```python
from build123d import *

# Parameters (mm, degrees)
F0_R           = 35.367098
F1_DEPTH       = 22.86
F2_D           = 20
F2_CBORE_D     = 22
F2_CBORE_DEPTH = 6.6
F3_R           = 10.89761
F4_DEPTH       = 6.604
F5_R           = 10.16


with BuildPart() as f1:
    # F0 (on Top) → F1 (new body)
    with BuildSketch(Plane.XY):
        Circle(F0_R)
    extrude(amount=F1_DEPTH)

    # F2 (through all)
    with Locations(Plane(origin=(0, 0, 0), x_dir=(1, 0, 0), z_dir=(0, 0, -1))):
        with Locations((0, 0)):
            CounterBoreHole(F2_D / 2, F2_CBORE_D / 2, F2_CBORE_DEPTH)

    # F3 (on face) → F4 (cut)
    with BuildSketch(Plane.XY.offset(22.86)):
        Circle(F3_R)
    extrude(amount=-F4_DEPTH, mode=Mode.SUBTRACT)

    # F5
    f5_edges = [f1.edges().sort_by_distance(p)[0] for p in [
        (35.367098, 0, 11.43),
        (-35.367098, 0, 0),
        (-35.367098, 0, 22.86),
    ]]
    fillet(f5_edges, radius=F5_R)


solid = f1.part
```
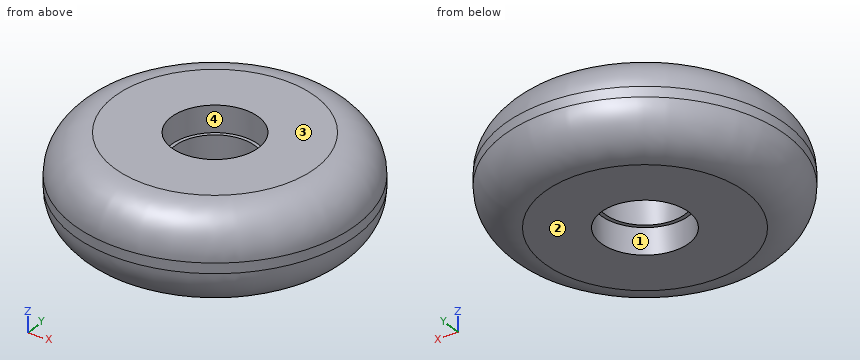
CAD build for the part. Positions are in the model's coordinates, mm. Face numbers are marked on the shaded views. A direction names the side the tool comes from. Coordinates: 2 decimals unless noted, no trailing zeros. Order: outer loops, then holes, each group sorted by start corner. A loop starts at its lowest first (then second) coordinate and runs counter-clockwise, first axis right, second up. Notation, with made-up numbers: (43, 76) - (63, 76) arc R8 cw to (63, 80) - close; hole circle Ø7 at (-7, 1.5). An arc over 180 degrees is marked (long way). Use a Markdown table: item, result. Add a question column.
(1) Saw through at A-A (x = 0). Give the cut face in (y, z), then the cut area to 3 significant figures.
(2) Saw through at D-D (z = 20.5). Give the cut face in (x, y).
(3) Drill centre lines: line 1 along Y through (x, z) = (0.5, 10.25); line 2 along Y through (x, z) = (0, 17.75); line 3 along X through (y, z) = (-7.5, 13). Where is each one in solid material? Low to high. Write a range as [from, to].
(4) Which spindle directions (+Z, -Z, +X, -X, +Y, -Y) get a long thin tool onto all of the face, cutting with end or side? Do the marked faces 3 and 4. Say none if no direction does.
(5) Saw through at C-C (z = 7.75). Give the cut face in (x, y).
(6) Pull direction Y, two halves, no side cores. Call the marked faces 1 and 2: +Y half, -Y half, draft (parallel to the pull), parting line (faces both ways), or undercut.
(7) Flat gauge pins, fed straight in: pin 1 (4 mm diameter, centred on y = -25.5, z = 14.5, fed in from +X); pin 2 (8 mm diameter, centred on y = -23.5, z = 10, fed in from -X); pin 3 (1 mm diameter, centred on x = 23.5, y = 21.5, fed in from -Z). Where does each tip first touch, or does it go through?
Solved:
| question | item | result |
|---|---|---|
| 1 | outline | (-35.37, 10.16) arc R10.16 ccw to (-25.21, 0) - (-11, 0) - (-11, 6.6) - (-10, 6.6) - (-10, 16.26) - (-10.9, 16.26) - (-10.9, 22.86) - (-25.21, 22.86) arc R10.16 ccw to (-35.37, 12.7) - close; (10, 6.6) - (11, 6.6) - (11, 0) - (25.21, 0) arc R10.16 ccw to (35.37, 10.16) - (35.37, 12.7) arc R10.16 ccw to (25.21, 22.86) - (10.9, 22.86) - (10.9, 16.26) - (10, 16.26) - close |
| 1 | area | 1,050 mm² |
| 2 | outline | circle Ø63.44 at (0, 0); hole circle Ø21.8 at (0, 0) |
| 3 | line 1 | y = [-35.36, -9.99], [9.99, 35.36] |
| 3 | line 2 | y = [-34.02, -10.9], [10.9, 34.02] |
| 3 | line 3 | x = [-34.56, -6.61], [6.61, 34.56] |
| 4 | face 3 | +Z, +X, -X, +Y, -Y |
| 4 | face 4 | +Z |
| 5 | outline | circle Ø70.15 at (0, 0); hole circle Ø20 at (0, 0) |
| 6 | face 1 | undercut |
| 6 | face 2 | draft |
| 7 | pin 1 | stops at x = 26.26 |
| 7 | pin 2 | stops at x = -29.5 |
| 7 | pin 3 | stops at z = 2.07 |
